Check sheet for the drawn part. Datum: minimum x, y, z corner. Units: mm. Coordinates: 2 decimals unless noted, no trailing zeros. Order: outer loops, then holes, each group sorted by start corner. A loop starts at its lowest first (then second) coordinate and runs counter-clockwise, first axis right, second up. Notation, with made-up numbers: M 44,36.5 L 80,36.5 A15 cw 80,54.5 Z; hole C 54.5,9 d11. An arc over 180 degrees is marked long. Use one line per item in the form item = value. Start each with the question number.
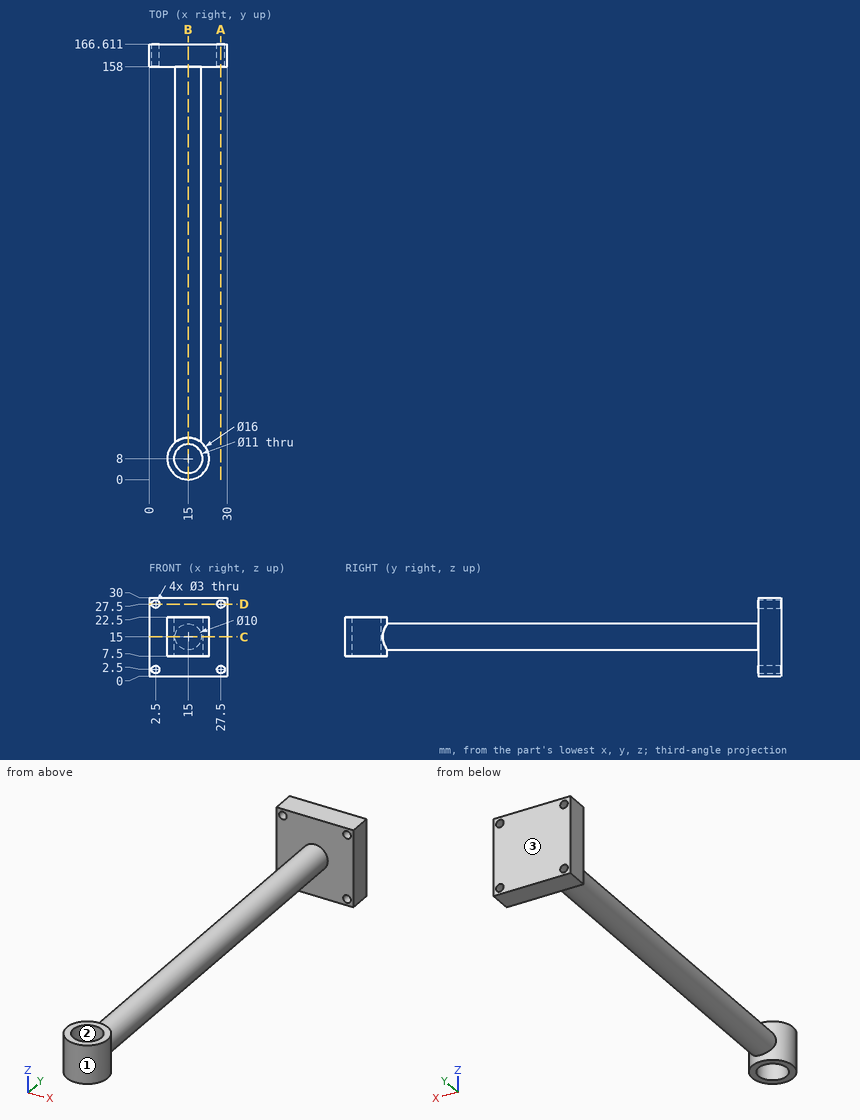
1. Release check for a two-part mould opening along Y. For the marked faces 1, 2 and 3 record: pulls with the +Y half, pulls with the -Y half, needs draft (parallel to the pull), parting line crosses it, or undercut.
2. Cross-section at C-C on z = 15. Enter the section's corners in (x, y) (3 decimals), and give its area (3 significant figures).
3. Material ranges on line 1 along X through (y, z) = (159.5, 2.5); line 2 along Y through (x, z) = (11.75, 21.25); line 3 along Y through (x, z) = (6.25, 12.5), recorded low to high.
4. Cross-section at A-A on x = 27.5. Enter the section's corners in (y, z), and give its area (3 significant figures).
5. Depth check by flat-ended pin: P1, Ø5, axis at x = 14, y = 80, coming from the -Z side; P2, Ø3.5, axis at x = 2.5, z = 2.5, coming from the -Y side; P3, Ø13, axis at x = 12, y = 8, coming from the +Z side. Enter the tip coordinate at first touch or a pass-through.
6. Cross-section at B-B on x = 15. Enter the section's corners in (y, z).
7. Cross-section at D-D on z = 27.5. Enter the section's corners in (x, y), and give its area (3 significant figures).
Final values:
q1.face_1 = undercut
q1.face_2 = undercut
q1.face_3 = pulls with the +Y half
q2.outline = M 0,158 L 10,158 L 10,14.245 A8 ccw long 20,14.245 L 20,158 L 30,158 L 30,166.611 L 0,166.611 Z; hole C 15,8 d11
q2.area = 1,790 mm2
q3.line_1 = 0 to 1, 4 to 26, 29 to 30
q3.line_2 = 0.69 to 3.56, 12.44 to 15.31, 158 to 166.61
q3.line_3 = 158 to 166.61
q4.outline = M 158,0 L 166.61,0 L 166.61,1 L 158,1 Z; M 158,4 L 166.61,4 L 166.61,26 L 158,26 Z; M 158,29 L 166.61,29 L 166.61,30 L 158,30 Z
q4.area = 207 mm2
q5.P1 = 10
q5.P2 = 158
q5.P3 = 22.5
q6.outline = M 0,7.5 L 2.5,7.5 L 2.5,22.5 L 0,22.5 Z; M 13.5,7.5 L 16,7.5 L 16,10 L 158,10 L 158,0 L 166.61,0 L 166.61,30 L 158,30 L 158,20 L 16,20 L 16,22.5 L 13.5,22.5 Z
q7.outline = M 0,158 L 1,158 L 1,166.61 L 0,166.61 Z; M 4,158 L 26,158 L 26,166.61 L 4,166.61 Z; M 29,158 L 30,158 L 30,166.61 L 29,166.61 Z
q7.area = 207 mm2
